The model under review builds one solid part; all positions refer to its coordinate system, in mm. Face numbers are marked on the shaded views. Round coordinates to 2 decimals unless told otherwise and drop trailing zeros. Write each loop counter-clockwise with the first axis right and the second up, starting at its lowest first coordinate (ties: lowest second). Pieces come first, ordered by that corner, then holes. Notation, with made-up numbers: (22, -16.5) -> (38, -16.5) arc R15 cw to (38, -0.5) -> close; hole circle Ø4 at (-6, -19.5). An arc over 180 degrees is marked (long way). Answer as a JSON object with one key per item and string values. Group by question number.
1) We need section D-D, the plane x = -27.5. Write out the cut boundary in (y, z) (3 decimals).
2) To check wall thickness, follow probe 1 along Y at (x, z) = (0, 13.5) (3 decimals); probe 2 along Y at (x, z) = (2, 6.25) (3 decimals); probe 3 along X at (y, z) = (-28.5, 3.75). State the ranges of each line that lie inside material, in increasing order. Write a range as [from, to].
3) We need section A-A, the plane x = 0. Write out the cut boundary in (y, z) (3 decimals).
4) Mouldability with a two-part tool opening along X and no side actions: class the marked faces 1, 2 and 3 as pulls with the +X half, pulls with the -X half, needs draft (parallel to the pull), parting line crosses it, or undercut.
5) We need section B-B, the plane y = 0. Write out the cut boundary in (x, z), then the cut area to 3 significant figures.
6) We need section C-C, the plane z = 6.25. Write out the cut boundary in (x, y) (3 decimals).
7) Insertion check: pin 1 Ø4.5 at (x, y) = (28.78, 0) entering from +Z. The pin has a flat end and moves straight along its axis. Give the tip position at first contact, or say it passes through.
from build123d import *

# Parameters (mm, degrees)
SKETCH2_W           = 107.95
SKETCH2_H           = 152.4
BOSS_EXTRUDE1_DEPTH = 19.558
SKETCH33_R          = 19.05
CUT_EXTRUDE4_DEPTH  = 96.405744004
SKETCH35_R          = 3.5814
CUT_EXTRUDE5_DEPTH  = 96.405744004


with BuildPart() as part:
    # Sketch2 → Boss-Extrude1 (new body)
    with BuildSketch(Plane(origin=(0, 0, 0), x_dir=(0, 1, 0), z_dir=(0, 0, 1))):
        Rectangle(SKETCH2_W, SKETCH2_H)
    extrude(amount=BOSS_EXTRUDE1_DEPTH)

    # Sketch33 → Cut-Extrude4 (cut, through all)
    with BuildSketch(Plane.XY.offset(19.558)):
        Circle(SKETCH33_R)
    extrude(amount=-CUT_EXTRUDE4_DEPTH, mode=Mode.SUBTRACT)

    # Sketch35 → Cut-Extrude5 (cut, through all)
    with BuildSketch(Plane.XY.offset(19.558)):
        with Locations((0, 28.7782)):
            Circle(SKETCH35_R)
        with Locations((28.7782, 0)):
            Circle(SKETCH35_R)
        with Locations((0, -28.7782)):
            Circle(SKETCH35_R)
        with Locations((-28.7782, 0)):
            Circle(SKETCH35_R)
    extrude(amount=-CUT_EXTRUDE5_DEPTH, mode=Mode.SUBTRACT)


solid = part.part
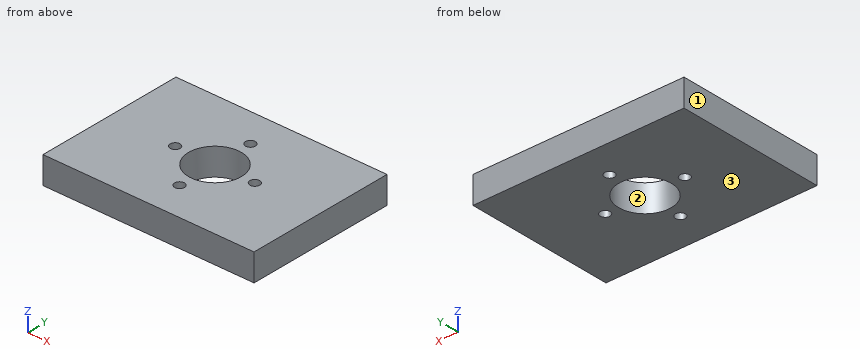
Here are the results:
{
 "1": {"outline": "(-53.975, 0) -> (-3.346, 0) -> (-3.346, 19.558) -> (-53.975, 19.558) -> close; (3.346, 0) -> (53.975, 0) -> (53.975, 19.558) -> (3.346, 19.558) -> close"},
 "2": {"probe 1": "y = [-53.975, -32.36], [-25.197, -19.05], [19.05, 25.197], [32.36, 53.975]", "probe 2": "y = [-53.975, -31.749], [-25.807, -18.945], [18.945, 25.807], [31.749, 53.975]", "probe 3": "x = [-76.2, -3.57], [3.57, 76.2]"},
 "3": {"outline": "(-53.975, 0) -> (-32.36, 0) -> (-32.36, 19.558) -> (-53.975, 19.558) -> close; (-25.197, 0) -> (-19.05, 0) -> (-19.05, 19.558) -> (-25.197, 19.558) -> close; (19.05, 0) -> (25.197, 0) -> (25.197, 19.558) -> (19.05, 19.558) -> close; (32.36, 0) -> (53.975, 0) -> (53.975, 19.558) -> (32.36, 19.558) -> close"},
 "4": {"face 1": "pulls with the -X half", "face 2": "undercut", "face 3": "needs draft"},
 "5": {"outline": "(-76.2, 0) -> (-32.36, 0) -> (-32.36, 19.56) -> (-76.2, 19.56) -> close; (-25.2, 0) -> (-19.05, 0) -> (-19.05, 19.56) -> (-25.2, 19.56) -> close; (19.05, 0) -> (25.2, 0) -> (25.2, 19.56) -> (19.05, 19.56) -> close; (32.36, 0) -> (76.2, 0) -> (76.2, 19.56) -> (32.36, 19.56) -> close", "area": "1,960 mm^2"},
 "6": {"outline": "(-76.2, -53.975) -> (76.2, -53.975) -> (76.2, 53.975) -> (-76.2, 53.975) -> close; hole circle Ø7.163 at (-28.778, 0); hole circle Ø38.1 at (0, 0); hole circle Ø7.163 at (0, -28.778); hole circle Ø7.163 at (0, 28.778); hole circle Ø7.163 at (28.778, 0)"},
 "7": {"pin 1": "passes through"}
}
